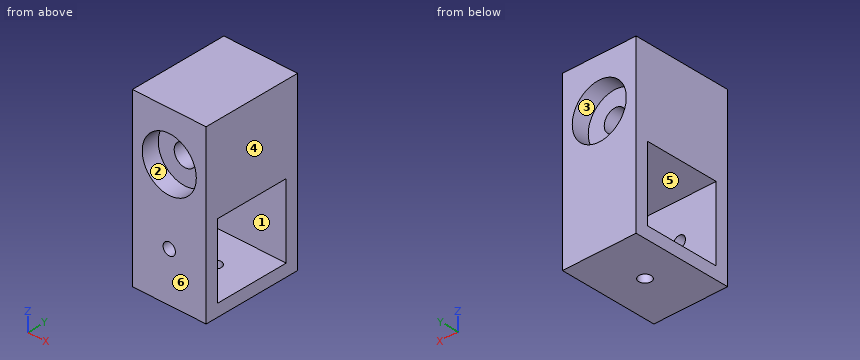
Autodesk Inventor part; units mm, degrees
ref_plane "YZ Plane" through (0, 0, 0) normal (1, 0, 0) x (0, 1, 0)
ref_plane "XZ Plane" through (0, 0, 0) normal (0, 1, 0) x (-1, 0, 0)
ref_plane "XY Plane" through (0, 0, 0) normal (0, 0, 1) x (1, 0, 0)
sketch "Sketch1" plane through (0, 0, 0) normal (0, 0, 1) x (1, 0, 0)
  line L0 (0, 0) -> (30, 0)
  line L1 (30, 0) -> (30, 40)
  line L2 (30, 40) -> (0, 40)
  line L3 (0, 40) -> (0, 0)
  dimension "d0" = 40
  dimension "d1" = 30
extrude "Extrusion1" add sketch "Sketch1" along normal blind 70
sketch "Sketch2" plane through (30, 0, 0) normal (1, 0, 0) x (0, 0, -1)
  line L0 (-5, 5) -> (-35, 5)
  line L1 (-35, 5) -> (-35, 35)
  line L2 (-35, 35) -> (-5, 35)
  line L3 (-5, 35) -> (-5, 5)
  line L4 (0, 0) -> (0, 40)
  line L5 (0, 0) -> (-70, 0)
  point P0 (-5, 20)
  dimension "d4" = 5
  dimension "d5" = 30
  dimension "d6" = 30
  dimension "d7" = 5
extrude "Extrusion2" cut sketch "Sketch2" against normal blind 70
sketch "Sketch3" plane through (0, 0, 0) normal (0, -1, 0) x (1, 0, 0)
  circle A0 centre (15, 50) radius 11
  line L0 (30, 35) -> (0, 35)
  line L1 (30, 0) -> (30, 70)
  point P0 (0, 0)
  dimension "d10" = 15
  dimension "d11" = 22
  dimension "d12" = 15
extrude "Extrusion3" cut sketch "Sketch3" against normal blind 7
sketch "Sketch4" plane through (0, 40, 0) normal (0, 1, 0) x (1, 0, 0)
  circle A0 centre (15, -50) radius 11
  line L0 (0, 0) -> (0, -70)
  point P0 (30, -35)
  dimension "d15" = 22
  dimension "d16" = 15
  dimension "d17" = 15
extrude "Extrusion4" cut sketch "Sketch4" against normal blind 7
sketch "Sketch5" plane through (15, 33, 50) normal (0, 1, 0) x (1, 0, 0)
  circle A0 centre (0, 0) radius 4.5
  point P0 (-15, 50)
  dimension "d20" = 9
extrude "Extrusion5" cut sketch "Sketch5" against normal blind 30
sketch "Sketch6" plane through (0, 0, 0) normal (0, -1, 0) x (1, 0, 0)
  circle A0 centre (15, 20) radius 2.5
  line L0 (0, 0) -> (0, 70)
  point P0 (0, 5)
  dimension "d23" = 5
  dimension "d24" = 15
  dimension "d25" = 15
extrude "Extrusion6" cut sketch "Sketch6" against normal blind 10
sketch "Sketch7" plane through (0, 0, 0) normal (0, 0, -1) x (-1, 0, 0)
  circle A0 centre (-15, 20) radius 2.5
  line L0 (0, 40) -> (0, 0)
  point P0 (0, 5)
  dimension "d28" = 5
  dimension "d29" = 15
  dimension "d30" = 15
extrude "Extrusion7" cut sketch "Sketch7" against normal blind 10
properties part number "double_gear_mount"
Design review of the part built by this model. Coordinates are the model's own, in mm. Face numbers are marked on the shaded views. A direction names the side the tool comes from. Coordinates: 2 decimals unless noted, no trailing zeros. Order: outer loops, then holes, each group sorted by start corner. A loop starts at its lowest first (then second) coordinate and runs counter-clockwise, first axis right, second up. Notation, with made-up numbers: M -30,64.5 L 19,64.5 A28 ccw 19,95.5 Z; hole C 73.25,44.25 d8. An arc over 180 degrees is marked long. Answer as a JSON object with one key per item and string values. Group by question number.
1) Add section C-C, the plane z = 50. Write out the cut boundary in (x, y), then the cut area to 3 significant figures.
2) For pin 1 (4 mm diameter, centred on x = 15, y = 20, fed in from -Z); pin 2 (1 mm diameter, centred on y = 27, z = 38, fed in from -X); pin 3 (10.5 mm diameter, centred on x = 15, z = 50, fed in from +Y); pin 4 (8 mm diameter, centred on x = 13, z = 51.5, fed in from -Y), all flat-tipped, find the tip position at first contact; note any pin that passes through.
3) Add section D-D, the plane y = 29. Write out the cut boundary in (x, z), then the cut area to 3 significant figures.
4) Add section A-A, the plane y = 18.5. Write out the cut boundary in (x, z).
5) Add section B-B, the plane x = 15. Write out the cut boundary in (y, z), then the cut area to 3 significant figures.
6) Tool access review of the marked faces 1, 2 and 3: name each direction out of +Z, -Z, +X, -X, +Y, -Y from which nothing blocks a thin tool from reaching the whole face with its end or side.
7) Wall thickness on L1, parallel to Z at x = 15, y = 3.5; L2, parallel to Y at x = 9.25, z = 11.5; L3, parallel to Z at x = 2, y = 13: over which ranges is each line inside the solid? List them lowest first.
8) Mouldability with a two-part tool opening along Y and no side actions: class the marked faces 4, 5 and 6 as pulls with the +Y half, pulls with the -Y half, needs draft (parallel to the pull), parting line crosses it, or undercut.
Computed values:
{
 "1": {"outline": "M 0,0 L 4,0 L 4,7 L 10.5,7 L 10.5,33 L 4,33 L 4,40 L 0,40 Z; M 19.5,7 L 26,7 L 26,0 L 30,0 L 30,40 L 26,40 L 26,33 L 19.5,33 Z", "area": "658 mm^2"},
 "2": {"pin 1": "stops at z = 35", "pin 2": "stops at x = 0", "pin 3": "stops at y = 33", "pin 4": "stops at y = 7"},
 "3": {"outline": "M 0,0 L 30,0 L 30,5 L 0,5 Z; M 0,35 L 30,35 L 30,70 L 0,70 Z; hole C 15,50 d9", "area": "1,140 mm^2"},
 "4": {"outline": "M 0,0 L 13,0 L 13,5 L 0,5 Z; M 0,35 L 30,35 L 30,70 L 0,70 Z; M 17,0 L 30,0 L 30,5 L 17,5 Z; hole C 15,50 d9"},
 "5": {"outline": "M 0,0 L 17.5,0 L 17.5,5 L 5,5 L 5,17.5 L 0,17.5 Z; M 0,22.5 L 5,22.5 L 5,35 L 35,35 L 35,5 L 22.5,5 L 22.5,0 L 40,0 L 40,39 L 33,39 L 33,45.5 L 7,45.5 L 7,39 L 0,39 Z; M 0,61 L 7,61 L 7,54.5 L 33,54.5 L 33,61 L 40,61 L 40,70 L 0,70 Z", "area": "1,310 mm^2"},
 "6": {"face 1": "+X, -X", "face 2": "-Y", "face 3": "+Y"},
 "7": {"L1": "z = 0 to 17.5, 22.5 to 39, 61 to 70", "L2": "y = 0 to 5, 35 to 40", "L3": "z = 0 to 5, 35 to 70"},
 "8": {"face 4": "needs draft", "face 5": "undercut", "face 6": "pulls with the -Y half"}
}
